Read the model definition and answer for the solid it produces. Units are mm, in the model's axes. Face numbers are marked on the shaded views. Round coordinates to 2 decimals unless told otherwise and drop trailing zeros. Write each loop counter-clockwise with the first axis right and the second up, starting at its lowest first coordinate (ties: lowest second). Pieces come first, ordered by that corner, then holes. Notation, with made-up numbers: (15.25, 50.5) -> (49.25, 50.5) arc R10 cw to (49.25, 60.5) -> close; hole circle Ø4 at (73.25, 83). An arc over 180 degrees is marked (long way). Return JSON: item names as keys, results as strings. Group by question number.
(1) The mould has two halves that part along X. Classify the marked faces 1, 2, 3 and 4: released by +X, released by -X, zero draft, split by the parting line, or undercut.
(2) A cutting plane is placed at A-A on z = 0. Give the vertices of the cut face in (x, y), then the cut area to 3 significant figures.
(3) A cutting plane is placed at C-C on x = 53. Give the vertices of the cut face in (y, z).
(4) A cutting plane is placed at D-D on z = 18.5. Give the vertices of the cut face in (x, y), then the cut area to 3 significant figures.
(5) Straight lines are drawn through the part: line 1 (X direction, y = -0.25, z = 0); line 2 (X direction, y = -0.7, z = 18.5); line 3 (Z direction, x = 76.5, y = -2.2). For each, find the intervals that lie inside material, in ascending order.
(6) Given pin 1 (5 mm diameter, centred on x = 75, z = 0, fed in from +Y); pin 2 (1.5 mm diameter, centred on y = 1, z = 1.5, fed in from +X); pin 3 (1.5 mm diameter, centred on y = 2, z = 16.5, fed in from +X), each flat-ended and moving along its own axis, determine where each tip first touches the part or whether it passes through.
(7) A cutting plane is placed at B-B on y = -0.4. Give the vertices of the cut face in (x, z).
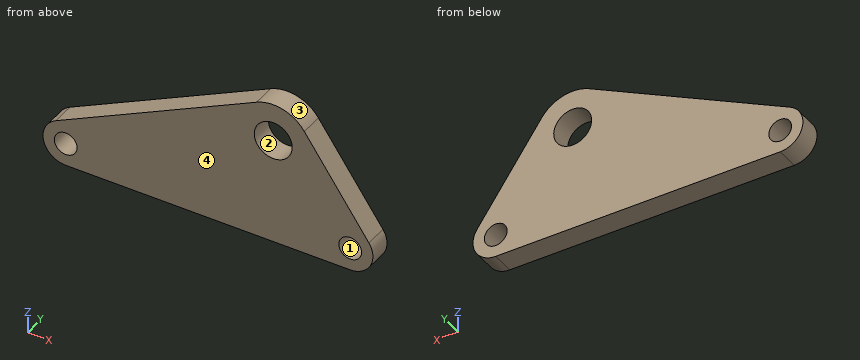
```python
from build123d import *

# Parameters (mm, degrees)
SKETCH_1_R      = 5
SKETCH_1_R_2    = 3
EXTRUDE_1_DEPTH = 3


with BuildPart() as part:
    # 草图1 → 凸台-拉伸1 (new, symmetric)
    with BuildSketch(Plane(origin=(0, 0, 0), x_dir=(1, 0, 0), z_dir=(0, 1, 0))):
        with BuildLine():
            Line((-2.618938967, -5.398255152), (50.341768388, -31.091901768))
            ThreePointArc((50.341768388, -31.091901768), (57.228686361, -31.77155603), (62.907769529, -27.816864709))
            Line((62.907769529, -27.816864709), (79.920661718, -3.433232917))
            ThreePointArc((79.920661718, -3.433232917), (80.319746117, 2.774941666), (75, 6))
            Line((75, 6), (0, 6))
            ThreePointArc((0, 6), (-5.847629046, 1.34359017), (-2.618938967, -5.398255152))
        make_face()
        with Locations(Location((54.706666667, -22.094809848, 0), (0, 0, 270))):
            Circle(SKETCH_1_R, mode=Mode.SUBTRACT)
        with Locations(Location((75, 0, 0), (0, 0, 270))):
            Circle(SKETCH_1_R_2, mode=Mode.SUBTRACT)
        with Locations(Location((0, 0, 0), (0, 0, 270))):
            Circle(SKETCH_1_R_2, mode=Mode.SUBTRACT)
    extrude(amount=EXTRUDE_1_DEPTH, both=True)


solid = part.part
```
Checks:
{
 "1": {"face 1": "undercut", "face 2": "undercut", "face 3": "split by the parting line", "face 4": "zero draft"},
 "2": {"outline": "(-6, -3) -> (-3, -3) -> (-3, 3) -> (-6, 3) -> close; (3, -3) -> (72, -3) -> (72, 3) -> (3, 3) -> close; (78, -3) -> (81, -3) -> (81, 3) -> (78, 3) -> close", "area": "450 mm^2"},
 "3": {"outline": "(-3, -6) -> (3, -6) -> (3, 17.4) -> (-3, 17.4) -> close; (-3, 26.79) -> (3, 26.79) -> (3, 31.95) -> (-3, 31.95) -> close"},
 "4": {"outline": "(24.39, -3) -> (51.23, -3) -> (51.23, 3) -> (24.39, 3) -> close; (58.18, -3) -> (69.41, -3) -> (69.41, 3) -> (58.18, 3) -> close", "area": "228 mm^2"},
 "5": {"line 1": "x = -6 to -3, 3 to 72, 78 to 81", "line 2": "x = 24.39 to 51.23, 58.18 to 69.41", "line 3": "z = -5.81 to -2.6, 2.6 to 8.34"},
 "6": {"pin 1": "passes through", "pin 2": "stops at x = 80.95", "pin 3": "stops at x = 71.33"},
 "7": {"outline": "(-2.62, 5.4) arc R6 ccw to (0, -6) -> (75, -6) arc R6 ccw to (79.92, 3.43) -> (62.91, 27.82) arc R10 ccw to (50.34, 31.09) -> close; hole circle Ø6 at (0, 0); hole circle Ø10 at (54.71, 22.09); hole circle Ø6 at (75, 0)"}
}
